```python
from build123d import *

# Parameters (mm, degrees)
ESBO_O1_R                = 28.62
RESSALTO_EXTRUS_O1_DEPTH = 11.11
ESBO_O2_R                = 17
RESSALTO_EXTRUS_O2_DEPTH = 39.95
ESBO_O3_R                = 10
CORTE_EXTRUS_O1_DEPTH    = 66.15621536
ESBO_O6_R                = 2.75
CORTE_EXTRUS_O3_DEPTH    = 11.11
CORTE_EXTRUS_O2_START    = 4.39
ESBO_O4_R                = 4.68
CORTE_EXTRUS_O2_DEPTH    = 53.480126604


with BuildPart() as part:
    # Esboço1 → Ressalto-extrusão1 (new body)
    with BuildSketch(Plane.XY):
        Circle(ESBO_O1_R)
    extrude(amount=RESSALTO_EXTRUS_O1_DEPTH)

    # Esboço2 → Ressalto-extrusão2 (add)
    with BuildSketch(Plane(origin=(0, 0, 0), x_dir=(-1, 0, 0), z_dir=(0, 0, -1))):
        with Locations(Location((0, 0, 0), (0, 0, 180))):
            Circle(ESBO_O2_R)
    extrude(amount=RESSALTO_EXTRUS_O2_DEPTH)

    # Esboço3 → Corte-extrusão1 (cut, through all)
    with BuildSketch(Plane(origin=(0, 0, -39.95), x_dir=(-1, 0, 0), z_dir=(0, 0, -1))):
        Circle(ESBO_O3_R)
    extrude(amount=-CORTE_EXTRUS_O1_DEPTH, mode=Mode.SUBTRACT)

    # Esboço6 → Corte-extrusão3 (cut)
    with BuildSketch(Plane.XY.offset(11.11)):
        with Locations((23.015, 0)):
            Circle(ESBO_O6_R)
        with Locations((11.5075, -19.931574668)):
            Circle(ESBO_O6_R)
        with Locations((-11.5075, -19.931574668)):
            Circle(ESBO_O6_R)
        with Locations((-23.015, 0)):
            Circle(ESBO_O6_R)
        with Locations((-11.5075, 19.931574668)):
            Circle(ESBO_O6_R)
        with Locations((11.5075, 19.931574668)):
            Circle(ESBO_O6_R)
    extrude(amount=-CORTE_EXTRUS_O3_DEPTH, mode=Mode.SUBTRACT)

    # Esboço4 → Corte-extrusão2 (cut, through all)
    with BuildSketch(Plane.XY.offset(CORTE_EXTRUS_O2_START)):
        with Locations((23.015, 0)):
            Circle(ESBO_O4_R)
        with Locations((11.5075, -19.931574668)):
            Circle(ESBO_O4_R)
        with Locations((-11.5075, -19.931574668)):
            Circle(ESBO_O4_R)
        with Locations((-23.015, 0)):
            Circle(ESBO_O4_R)
        with Locations((-11.5075, 19.931574668)):
            Circle(ESBO_O4_R)
        with Locations((11.5075, 19.931574668)):
            Circle(ESBO_O4_R)
    extrude(amount=CORTE_EXTRUS_O2_DEPTH, mode=Mode.SUBTRACT)


solid = part.part
```
The model under review builds one solid part; all positions refer to its coordinate system, in mm. A direction names the side the tool comes from. Round coordinates to 2 decimals unless told otherwise and drop trailing zeros. Order: outer loops, then holes, each group sorted by start corner. A loop starts at its lowest first (then second) coordinate and runs counter-clockwise, first axis right, second up.
Item 1: Draft analysis for pull direction X (two halves, no side actions). For faces 3 (the flat face through (12.3, -12.3, 0)), 4 (the cylindrical face through (-2.213, -16.855, -19.695)), 5 (the cylindrical face through (-11.865, -17.205, 2.226)), state which applies: released by +X, released by -X, zero draft, split by the parting line, or undercut.
Working result:
face 3: zero draft
face 4: split by the parting line
face 5: undercut
Item 2: Add section D-D, the plane z = 6.5. State the section outline as (x, y) points (1 decimal), and give its area (3 significant figures).
Working result:
outline: circle Ø57.2 at (0, 0); hole circle Ø9.4 at (-23, 0); hole circle Ø9.4 at (-11.5, -19.9); hole circle Ø9.4 at (-11.5, 19.9); hole circle Ø20 at (0, 0); hole circle Ø9.4 at (11.5, -19.9); hole circle Ø9.4 at (11.5, 19.9); hole circle Ø9.4 at (23, 0)
area: 1,850 mm2
Item 3: Machinability: for faces 1 (the cylindrical face through (-20.392, 0.826, 2.226)), 2 (the cylindrical face through (-8.992, 23.878, 7.703)), which of the approach directions +Z, -Z, +X, -X, +Y, -Y give a long, thin tool a straight path to every point of the face, cutting with its end or side? Answer none if there is none.
Working result:
face 1: +Z, -Z
face 2: +Z
Item 4: For pin 1 (4 mm diameter, centred on y = 2.5, z = -6, fed in from +X); pin 2 (7.5 mm diameter, centred on x = -11.51, y = 19.93, fed in from -Z); pin 3 (3 mm diameter, centred on x = 10.5, y = 22, fed in from +Z); pin 4 (3.5 mm diameter, centred on x = 23.015, y = 0, fed in from -Z), all flat-tipped, find the tip position at first contact; note any pin that passes through.
Working result:
pin 1: stops at x = 16.99
pin 2: stops at z = 0
pin 3: stops at z = 4.39
pin 4: passes through
Item 5: To check wall thickness, follow probe 1 along X at (y, z) = (-0.5, -22); probe 2 along Y at (x, z) = (0, -26); probe 3 along Z at (x, y) = (-9, -25.5). State the ranges of each line that lie inside material, in increasing order.
Working result:
probe 1: x = -16.99 to -9.99, 9.99 to 16.99
probe 2: y = -17 to -10, 10 to 17
probe 3: z = 0 to 11.11
Item 6: Add section C-C, the plane y = 19. State the section outline as (x, z) points.
Working result:
outline: (-21.4, 0) - (-14.09, 0) - (-14.09, 4.39) - (-16.09, 4.39) - (-16.09, 11.11) - (-21.4, 11.11) - close; (-8.92, 0) - (8.92, 0) - (8.92, 4.39) - (6.92, 4.39) - (6.92, 11.11) - (-6.92, 11.11) - (-6.92, 4.39) - (-8.92, 4.39) - close; (14.09, 0) - (21.4, 0) - (21.4, 11.11) - (16.09, 11.11) - (16.09, 4.39) - (14.09, 4.39) - close
Item 7: Add section B-B, the plane y = 0. State the section outline as (x, z) points (3 decimals), and give its area (3 significant figures).
Working result:
outline: (-28.62, 0) - (-25.765, 0) - (-25.765, 4.39) - (-27.695, 4.39) - (-27.695, 11.11) - (-28.62, 11.11) - close; (-20.265, 0) - (-17, 0) - (-17, -39.95) - (-10, -39.95) - (-10, 11.11) - (-18.335, 11.11) - (-18.335, 4.39) - (-20.265, 4.39) - close; (10, -39.95) - (17, -39.95) - (17, 0) - (20.265, 0) - (20.265, 4.39) - (18.335, 4.39) - (18.335, 11.11) - (10, 11.11) - close; (25.765, 0) - (28.62, 0) - (28.62, 11.11) - (27.695, 11.11) - (27.695, 4.39) - (25.765, 4.39) - close
area: 799 mm2
Item 8: Add section A-A, the plane x = 0. State the section outline as (y, z) points.
Working result:
outline: (-28.62, 0) - (-17, 0) - (-17, -39.95) - (-10, -39.95) - (-10, 11.11) - (-28.62, 11.11) - close; (10, -39.95) - (17, -39.95) - (17, 0) - (28.62, 0) - (28.62, 11.11) - (10, 11.11) - close
